Drawing for the job (mm, zero at the part's lowest x, y, z). Give positions to 0.01 mm unless a question says otherwise; leave off trailing zeros. Order: outer loops, then holes, each group sorted by start corner. A loop starts at its lowest first (then second) coordinate and runs counter-clockwise, first axis right, second up. Notation, with made-up numbers: (74.5, 45.25) - (103.5, 45.25) arc R27 ccw to (103.5, 78.25) - close; hole circle Ø10 at (74.5, 44). An arc over 180 degrees is marked (long way). Write each question's results on one line, items separated by ' | '. Start each with the question number.
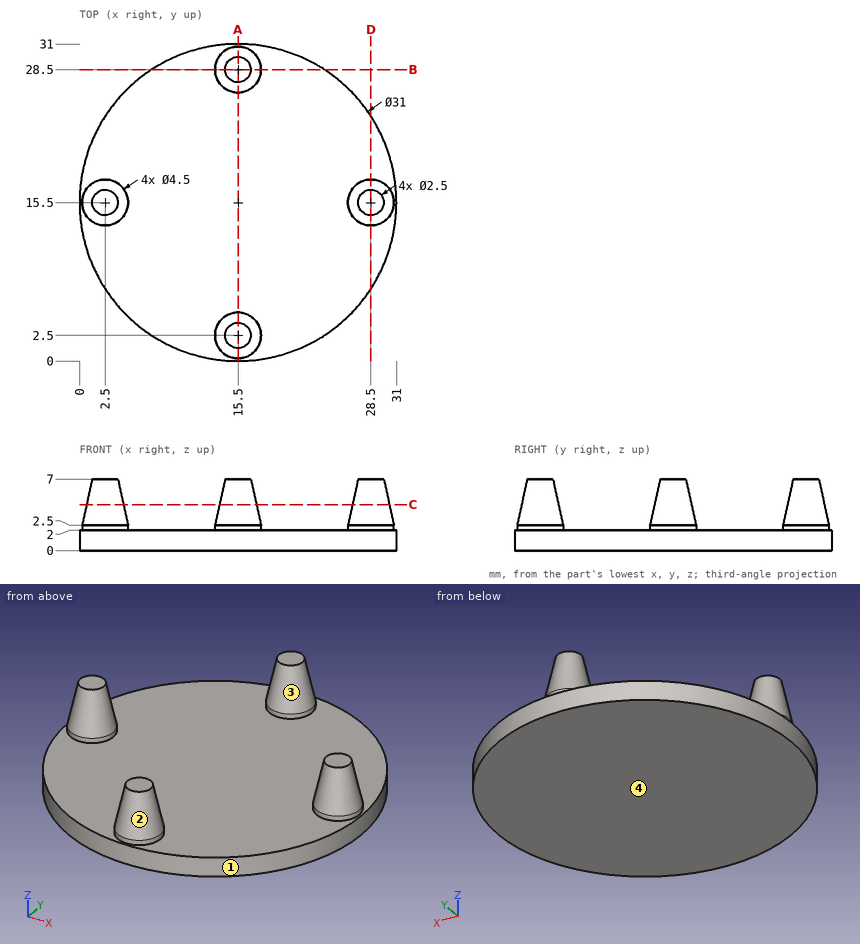
Item 1: Flat gauge pins, fed straight in: pin 1 Ø5 at (x, y) = (20.5, 9) entering from +Z; pin 2 Ø4 at (x, z) = (3.5, 1.5) entering from +Y; pin 3 Ø8 at (x, y) = (20.5, 6.5) entering from -Z; pin 4 Ø1.5 at (y, z) = (13.5, 3.5) entering from +X. Where does each tip first touch, or does it go through?
Item 2: Cut at B-B, the plane y = 28.5. List the corners of the cut face in (x, z), then the cut area to 3 significant figures.
Item 3: Cut at A-A, the plane x = 15.5. List the corners of the cut face in (y, z), then the cut area to 3 significant figures.
Item 4: Cut at C-C, the plane z = 4.5. List the corners of the cut face in (x, y).
Item 5: Two-plate mould, pull along Y, no slides. Class the marked faces 1, 2, 3 and 4: +Y half, -Y half, draft (parallel to the pull), parting line (faces both ways), or undercut.
Item 6: Probe line 1 along Y through (x, z) = (15.5, 2.25); line 2 along Z through (x, y) = (12, 20); line 3 along X through (y, z) = (6.5, 1.75). List the from-to ranges inside material, lowest first. Write a range as from..to.
Values found:
1) pin 1: stops at z = 2 | pin 2: stops at y = 27.34 | pin 3: stops at z = 0 | pin 4: stops at x = 30.13
2) outline: (7.06, 0) - (23.94, 0) - (23.94, 2) - (17.75, 2) - (17.75, 2.5) - (16.75, 7) - (14.25, 7) - (13.25, 2.5) - (13.25, 2) - (7.06, 2) - close | area: 51.8 mm2
3) outline: (0, 0) - (31, 0) - (31, 2) - (30.75, 2) - (30.75, 2.5) - (29.75, 7) - (27.25, 7) - (26.25, 2.5) - (26.25, 2) - (4.75, 2) - (4.75, 2.5) - (3.75, 7) - (1.25, 7) - (0.25, 2.5) - (0.25, 2) - (0, 2) - close | area: 98.0 mm2
4) outline: circle Ø3.61 at (2.5, 15.5); circle Ø3.61 at (15.5, 2.5); circle Ø3.61 at (15.5, 28.5); circle Ø3.61 at (28.5, 15.5)
5) face 1: parting line | face 2: undercut | face 3: undercut | face 4: draft
6) line 1: y = 0.25..4.75, 26.25..30.75 | line 2: z = 0..2 | line 3: x = 2.88..28.12
